The listing builds one solid part. Answer for the finished solid, in the listing's coordinates (mm). Round coordinates to 2 decimals unless told otherwise and drop trailing zeros. Write each loop counter-clockwise with the first axis right and the second up, starting at its lowest first coordinate (ties: lowest second). Pieces come first, ordered by that corner, then holes. Notation, with made-up numbers: (43, 58) - (69, 58) arc R14 ccw to (69, 69) - close; hole circle Ø1 at (34, 29). An arc over 180 degrees is marked (long way). Answer in a Markdown table with one row per item.
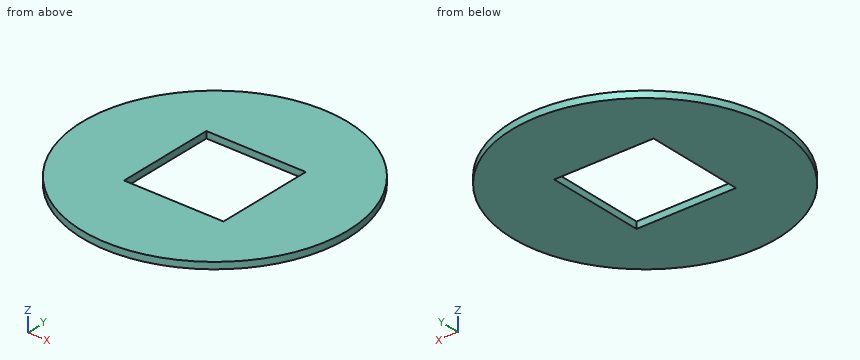
from build123d import *

# Parameters (mm, degrees)
SKETCH1_R           = 10
BOSS_EXTRUDE1_DEPTH = 0.5
SKETCH2_W           = 7.5
SKETCH2_H           = 7.5
BOSS_EXTRUDE2_DEPTH = 0.5
SKETCH3_W           = 7.5
SKETCH3_H           = 7.5
CUT_EXTRUDE1_DEPTH  = 15.150971698


with BuildPart() as part:
    # Sketch1 → Boss-Extrude1 (new body)
    with BuildSketch(Plane.XY):
        Circle(SKETCH1_R)
    extrude(amount=BOSS_EXTRUDE1_DEPTH)

    # Sketch2 → Boss-Extrude2 (add, through all)
    with BuildSketch(Plane.XY.offset(0.5)):
        Rectangle(SKETCH2_W, SKETCH2_H)
    extrude(amount=-BOSS_EXTRUDE2_DEPTH)

    # Sketch3 → Cut-Extrude1 (cut, through all)
    with BuildSketch(Plane.XY.offset(0.5)):
        Rectangle(SKETCH3_W, SKETCH3_H)
    extrude(amount=-CUT_EXTRUDE1_DEPTH, mode=Mode.SUBTRACT)


solid = part.part
(1) Section C-C (z = 0.3) is taken. Give the vertices of the cut face in (x, y), and give its area (3 significant figures).
Checked values:
| item | result |
|---|---|
| outline | circle Ø20 at (0, 0); hole (-3.75, -3.75) - (3.75, -3.75) - (3.75, 3.75) - (-3.75, 3.75) - close |
| area | 258 mm2 |
(2) Section A-A (y = 0) is taken. Give the vertices of the cut face in (x, z), and give its area (3 significant figures).
Checked values:
| item | result |
|---|---|
| outline | (-10, 0) - (-3.75, 0) - (-3.75, 0.5) - (-10, 0.5) - close; (3.75, 0) - (10, 0) - (10, 0.5) - (3.75, 0.5) - close |
| area | 6.25 mm2 |
(3) Find the intervals of material crossed by line 1 (X direction, y = 0.25, z = 0.3); line 2 (Y direction, x = 0.5, z = 0.45); line 3 (Y direction, x = 3.5, z = 0.2), in increasing order.
Checked values:
| item | result |
|---|---|
| line 1 | x = -10 to -3.75, 3.75 to 10 |
| line 2 | y = -9.99 to -3.75, 3.75 to 9.99 |
| line 3 | y = -9.37 to -3.75, 3.75 to 9.37 |
(4) A flat-ended cylindrical pin translates along its axis: pin 1 (2 mm diameter, centred on x = -4, y = 2, fed in from -Z). Find the tip coordinate at first contact, or state that the pin passes through.
Checked values:
| item | result |
|---|---|
| pin 1 | stops at z = 0 |
(5) Section D-D (x = 5.75) is taken. Give the vertices of the cut face in (y, z).
Checked values:
| item | result |
|---|---|
| outline | (-8.18, 0) - (8.18, 0) - (8.18, 0.5) - (-8.18, 0.5) - close |
